Work out the finished part from the listing and answer in its coordinate system (mm). Face numbers are marked on the shaded views. A direction names the side the tool comes from. Round coordinates to 2 decimals unless told otherwise and drop trailing zeros. Write each loop counter-clockwise with the first axis right and the second up, starting at its lowest first coordinate (ties: lowest second). Pieces come first, ordered by that corner, then holes. Notation, with made-up numbers: (8.25, 11.5) -> (60.25, 11.5) arc R21 cw to (60.25, 44.5) -> close; hole circle Ø10 at (-0.75, 18.25). An arc over 180 degrees is marked (long way). One line per item, written item: value.
```python
from build123d import *

# Parameters (mm, degrees)
SKETCH_R     = 1.65
PAD_DEPTH    = 5
SKETCH001_W  = 10
SKETCH001_H  = 30
PAD001_DEPTH = 10
SKETCH002_R  = 1.5
POCKET_DEPTH = 15


with BuildPart() as part:
    # Sketch → Pad (new body)
    with BuildSketch(Plane.XY):
        Polygon((-23, 21), (23, 21), (23, 13.5), (16, 13.5), (16, -1.5), (23, -1.5), (23, -22), (-23, -22), align=None)
        with Locations((-19.5, 18)):
            Circle(SKETCH_R, mode=Mode.SUBTRACT)
        with Locations((19.5, 18)):
            Circle(SKETCH_R, mode=Mode.SUBTRACT)
        with Locations((-19.5, -19)):
            Circle(SKETCH_R, mode=Mode.SUBTRACT)
        with Locations((19.5, -19)):
            Circle(SKETCH_R, mode=Mode.SUBTRACT)
    extrude(amount=-PAD_DEPTH)

    # Sketch001 (on Face14 of Pad) → Pad001 (join)
    with BuildSketch(Plane(origin=(0, 0, -5), x_dir=(1, 0, 0), z_dir=(0, 0, -1))):
        with Locations((10, -6)):
            Rectangle(SKETCH001_W, SKETCH001_H)
    extrude(amount=PAD001_DEPTH)

    # Sketch002 (on Face17 of Pad001) → Pocket (cut)
    with BuildSketch(Plane(origin=(0, 0, -15), x_dir=(1, 0, 0), z_dir=(0, 0, -1))):
        with Locations((10, 6)):
            Circle(SKETCH002_R)
        with Locations((10, -18)):
            Circle(SKETCH002_R)
    extrude(amount=-POCKET_DEPTH, mode=Mode.SUBTRACT)


solid = part.part
```
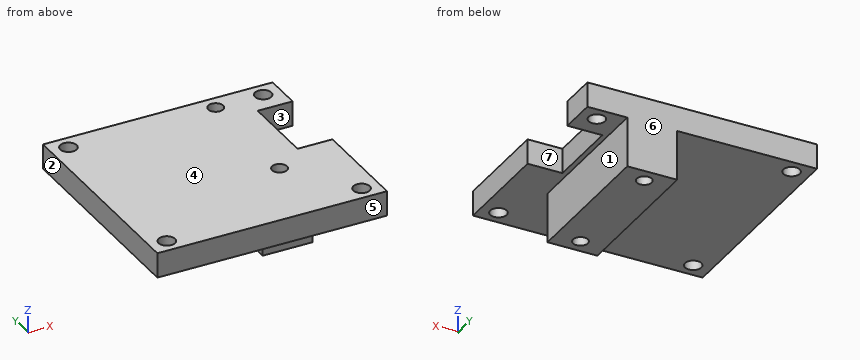
(1) Find section B-B on y = -6. Give the vertices of the cut face in (x, z), plus the area to 3 significant figures.
Reported:
outline: (-23, -5) -> (5, -5) -> (5, -15) -> (8.5, -15) -> (8.5, 0) -> (-23, 0) -> close; (11.5, -15) -> (15, -15) -> (15, -5) -> (23, -5) -> (23, 0) -> (11.5, 0) -> close
area: 285 mm2
(2) Find section A-A on x = 10. Give the vertices of the cut face in (y, z), plus the area to 3 significant figures.
Reported:
outline: (-22, -5) -> (-9, -5) -> (-9, -15) -> (-7.5, -15) -> (-7.5, 0) -> (-22, 0) -> close; (-4.5, -15) -> (16.5, -15) -> (16.5, 0) -> (-4.5, 0) -> close; (19.5, -15) -> (21, -15) -> (21, 0) -> (19.5, 0) -> close
area: 425 mm2
(3) Flat-ended cylindrical pins translate along their axes: pin 1 Ø1 at (x, y) = (-8.5, 1) entering from -Z; pin 2 Ø8 at (x, z) = (2, -8.5) entering from -Y; pin 3 Ø3 at (x, z) = (11.5, -11) entering from -Y; pin 4 Ø1.5 at (y, z) = (9.5, -3.5) entering from +X. Find the tip coordinate at first contact, or state that the pin passes through.
Reported:
pin 1: stops at z = -5
pin 2: stops at y = -22
pin 3: stops at y = -9
pin 4: stops at x = 16
(4) Find section D-D on z = -6. Give the vertices of the cut face in (x, y), plus the area to 3 significant figures.
Reported:
outline: (5, -9) -> (15, -9) -> (15, 21) -> (5, 21) -> close; hole circle Ø3 at (10, -6); hole circle Ø3 at (10, 18)
area: 286 mm2
(5) Find section C-C on y = -19. Give the vertices of the cut face in (x, z).
Reported:
outline: (-23, -5) -> (-21.15, -5) -> (-21.15, 0) -> (-23, 0) -> close; (-17.85, -5) -> (17.85, -5) -> (17.85, 0) -> (-17.85, 0) -> close; (21.15, -5) -> (23, -5) -> (23, 0) -> (21.15, 0) -> close
(6) Consider probe 1 along Y at (x, z) = (10, -4.75); probe 2 along Y at (x, z) = (19.5, -1.35); probe 3 along Y at (x, z) = (-19.5, -1.8). Determine where each line is inside the solid, lowest interval first.
Reported:
probe 1: y = -22 to -7.5, -4.5 to 16.5, 19.5 to 21
probe 2: y = -22 to -20.65, -17.35 to -1.5, 13.5 to 16.35, 19.65 to 21
probe 3: y = -22 to -20.65, -17.35 to 16.35, 19.65 to 21
(7) A tool of negligible diameter and unlimited length cuts with its end or side. For the marked faces 1, 2 and 3, from which of +Z, -Z, +X, -X, +Y, -Y can it reach the whole face along a straight path? Write none if from no direction.
Reported:
face 1: -Z, +X, +Y, -Y
face 2: +Z, -Z, -X, +Y, -Y
face 3: +Z, -Z, +X
(8) For a pull along Y with two mould halves and no side action, classify the marked faces 4, 5, 6 and 7 as pulls with the +Y half, pulls with the -Y half, needs draft (parallel to the pull), parting line crosses it, or undercut.
Reported:
face 4: needs draft
face 5: pulls with the -Y half
face 6: pulls with the +Y half
face 7: undercut
